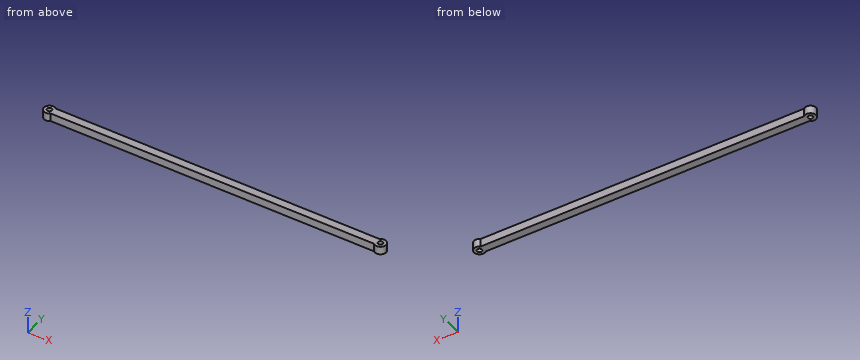
from build123d import *

# Parameters (mm, degrees)
BOSS_EXTRUDE1_DEPTH             = 290.957
BOSS_EXTRUDE1_DEPTH_BACK        = 290.957
SKETCH3_W                       = 13.97
SKETCH3_H                       = 13.97
BOSS_EXTRUDE4_REACH             = 293.125
SKETCH6_R                       = 9.525
BOSS_EXTRUDE4_DIRECTION_2_REACH = 293.125
SKETCH7_R                       = 4.191
CUT_EXTRUDE2_DEPTH              = 301.714063811


with BuildPart() as part:
    # Sketch3 → Boss-Extrude1 (new, two sides: drawn at the far end of the back side and taken through both)
    with BuildSketch(Plane(origin=(0, 0, 0), x_dir=(0, 0, -1), z_dir=(1, 0, 0)).offset(-BOSS_EXTRUDE1_DEPTH_BACK)):
        Rectangle(SKETCH3_W, SKETCH3_H)
    extrude(amount=BOSS_EXTRUDE1_DEPTH + BOSS_EXTRUDE1_DEPTH_BACK)

    # Boss-Extrude4: up to this face of the body (flat: up to its plane)
    boss_extrude4_end = Plane(part.part.faces().sort_by_distance((0, 0, -6.985))[0])
    # Sketch6 → Boss-Extrude4 (add, up to the picked face)
    with BuildSketch(Plane.XY, mode=Mode.PRIVATE) as boss_extrude4_sk1:
        with Locations((290.957, 0)):
            Circle(SKETCH6_R)
    boss_extrude4_tool1 = split(extrude(boss_extrude4_sk1.sketch, amount=-BOSS_EXTRUDE4_REACH, mode=Mode.PRIVATE), bisect_by=boss_extrude4_end, keep=Keep.BOTH, mode=Mode.PRIVATE)
    boss_extrude4 = boss_extrude4_tool1.solids().sort_by(Axis((290.957, 0, 0), (0, 0, -1)))[0]
    add(boss_extrude4)

    # Boss-Extrude4 direction 2: up to this face of the body (flat: up to its plane)
    boss_extrude4_direction_2_end = Plane(part.part.faces().sort_by_distance((0, 0, 6.985))[0])
    # Sketch6 → Boss-Extrude4 direction 2 (add, up to the picked face)
    with BuildSketch(Plane.XY, mode=Mode.PRIVATE) as boss_extrude4_direction_2_sk1:
        with Locations((290.957, 0)):
            Circle(SKETCH6_R)
    boss_extrude4_direction_2_tool1 = split(extrude(boss_extrude4_direction_2_sk1.sketch, amount=BOSS_EXTRUDE4_DIRECTION_2_REACH, mode=Mode.PRIVATE), bisect_by=boss_extrude4_direction_2_end, keep=Keep.BOTH, mode=Mode.PRIVATE)
    boss_extrude4_direction_2 = boss_extrude4_direction_2_tool1.solids().sort_by(Axis((290.957, 0, 0), (0, 0, 1)))[0]
    add(boss_extrude4_direction_2)

    # Sketch7 → Cut-Extrude2 (cut, symmetric)
    with BuildSketch(Plane.XY):
        with Locations((290.957, 0)):
            Circle(SKETCH7_R)
    cut_extrude2 = extrude(amount=CUT_EXTRUDE2_DEPTH, both=True, mode=Mode.SUBTRACT)

    # Mirror3: Boss-Extrude4, Boss-Extrude4 direction 2, Cut-Extrude2 across plane
    add(boss_extrude4.mirror(Plane(origin=(0, 0, 0), x_dir=(0, 0, 1), z_dir=(1, 0, 0))))
    add(boss_extrude4_direction_2.mirror(Plane(origin=(0, 0, 0), x_dir=(0, 0, 1), z_dir=(1, 0, 0))))
    add(cut_extrude2.mirror(Plane(origin=(0, 0, 0), x_dir=(0, 0, 1), z_dir=(1, 0, 0))), mode=Mode.SUBTRACT)


solid = part.part
Design review of the part built by this model. Coordinates are the model's own, in mm. Round coordinates to 2 decimals unless told otherwise and drop trailing zeros. Write each loop counter-clockwise with the first axis right and the second up, starting at its lowest first coordinate (ties: lowest second). Pieces come first, ordered by that corner, then holes.
Item 1: Consider section A-A on z = -0.5. Give the boundary of the cut face in (x, y) (3 decimals), and give its area (3 significant figures).
Item 2: Consider section C-C on x = -206. Give the boundary of the cut face in (y, z) (3 decimals), and give its area (3 significant figures).
Item 3: Wall thickness on L1, parallel to X at y = 1.5, z = -3; L2, parallel to X at y = -2, z = 5.25; L3, parallel to Y at x = 207.5, z = 1 (3 decimals): over which ranges is each line inside the solid? List them lowest first.
Item 4: For pin 1 Ø4 at (x, z) = (9, 0) entering from +Y (3 decimals); pin 2 Ø6 at (y, z) = (3.5, 5.5) entering from -X; pin 3 Ø4 at (y, z) = (5.5, 3.5) entering from +X; pin 4 Ø7.5 at (x, y) = (290.957, 0) entering from +Z, all flat-tipped, find the tip position at first contact; note any pin that passes through.
Item 5: Consider section B-B on y = 0. Give the boundary of the cut face in (x, z) (3 decimals), and give its area (3 significant figures).
Check values:
1. outline: (-284.481, -6.985) - (284.481, -6.985) arc R9.525 ccw (long way) to (284.481, 6.985) - (-284.481, 6.985) arc R9.525 ccw (long way) to start; hole circle Ø8.382 at (-290.957, 0); hole circle Ø8.382 at (290.957, 0)
1. area: 8,350 mm2
2. outline: (-6.985, -6.985) - (6.985, -6.985) - (6.985, 6.985) - (-6.985, 6.985) - close
2. area: 195 mm2
3. L1: x = -300.36 to -294.87, -287.04 to 287.04, 294.87 to 300.36
3. L2: x = -300.27 to -294.64, -287.27 to 287.27, 294.64 to 300.27
3. L3: y = -6.985 to 6.985
4. pin 1: stops at y = 6.985
4. pin 2: stops at x = -300.47
4. pin 3: stops at x = 299.82
4. pin 4: passes through
5. outline: (-300.482, -6.985) - (-295.148, -6.985) - (-295.148, 6.985) - (-300.482, 6.985) - close; (-286.766, -6.985) - (286.766, -6.985) - (286.766, 6.985) - (-286.766, 6.985) - close; (295.148, -6.985) - (300.482, -6.985) - (300.482, 6.985) - (295.148, 6.985) - close
5. area: 8,160 mm2
